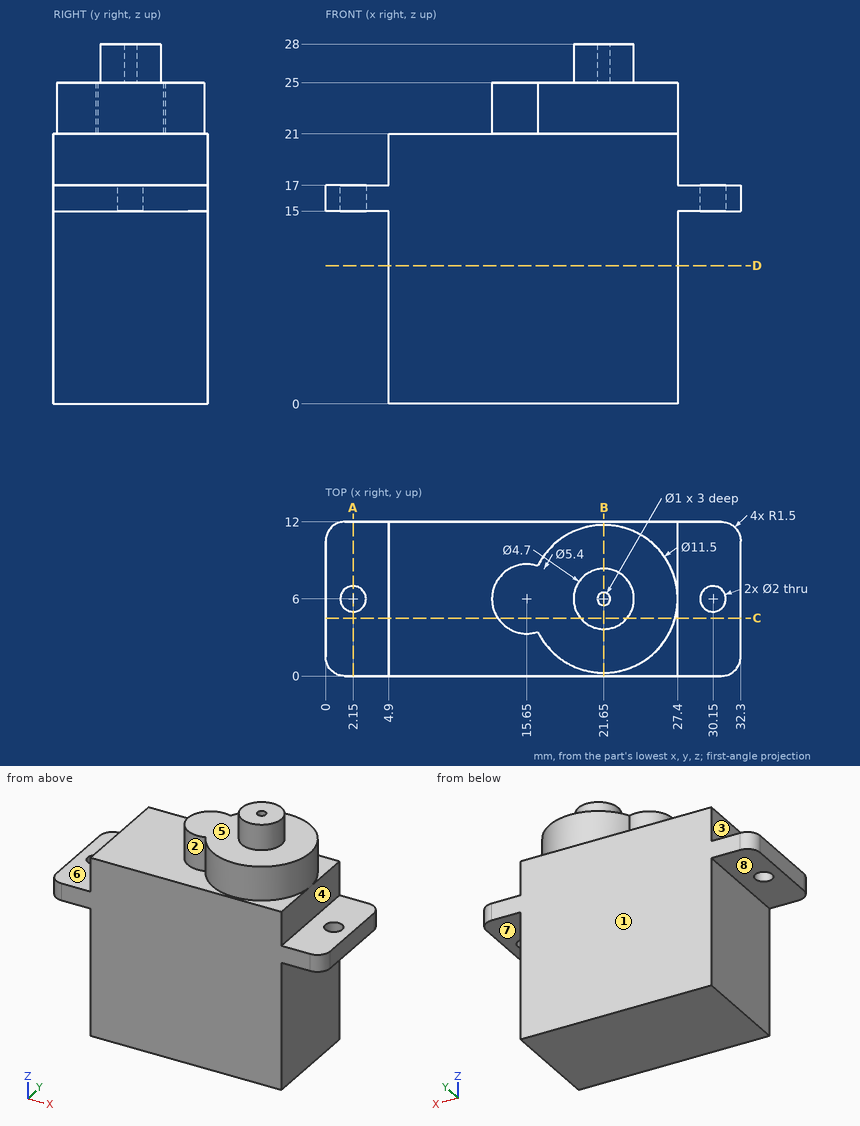
For this review, use the dimensioned drawing (mm, ordinates from the lowest corner) and the shaded views. A direction names the side the tool comes from. Give positions to 0.01 mm unless a question says otherwise; leave off trailing zeros. Write each loop counter-clockwise with the first axis right and the second up, starting at its lowest first coordinate (ties: lowest second). Pieces come first, ordered by that corner, then holes. Notation, with made-up numbers: M 31.25,28 L 69.25,28 A30 cw 69.25,64 Z; hole C 12,88.25 d8. An arc over 180 degrees is marked long. Answer as a JSON object with one key per item and string values. Group by question number.
1) We need section D-D (z = 10.75). Give the boundary of the cut face in (x, y), and give its area (3 significant figures).
2) Mouldability with a two-part tool opening along X and no side actions: class the marked faces 1, 2 and 3 as released by +X, released by -X, zero draft, split by the parting line, or undercut.
3) Clearance check with flat-ended pins moving along their axes: pin 1 Ø4 at (x, z) = (10.5, 8.5) entering from -Y; pin 2 Ø6 at (y, z) = (9, 7) entering from +X; pin 3 Ø3 at (y, z) = (8.5, 19) entering from -X; pin 4 Ø5 at (x, y) = (6, 7.5) entering from +Z. State where each tip first meets the part, or that it passes through.
4) Tool access review of the marked faces 4, 5, 6, 7 and 8: name each direction out of +Z, -Z, +X, -X, +Y, -Y from which nothing blocks a thin tool from reaching the whole face with its end or side.
5) We need section C-C (y = 4.5). Give the boundary of the cut face in (x, z) (3 decimals), and give its area (3 significant figures).
6) For line 1 along Y through (x, z) = (2.15, 15.6); line 2 along Y through (x, z) = (21.65, 25.9); line 3 along X through (y, z) = (4, 10.5), list the stretches that pass through material, from the lowest coordinate up.
7) We need section A-A (x = 2.15). Give the boundary of the cut face in (y, z), and give its area (3 significant figures).
8) We need section B-B (x = 21.65). Give the boundary of the cut face in (y, z), and give its area (3 significant figures).
Answer key:
{
 "1": {"outline": "M 4.9,0 L 27.4,0 L 27.4,12 L 4.9,12 Z", "area": "270 mm²"},
 "2": {"face 1": "zero draft", "face 2": "undercut", "face 3": "released by -X"},
 "3": {"pin 1": "stops at y = 0", "pin 2": "stops at x = 27.4", "pin 3": "stops at x = 4.9", "pin 4": "stops at z = 21"},
 "4": {"face 4": "+Z, +X, +Y, -Y", "face 5": "+Z", "face 6": "+Z, -X, +Y, -Y", "face 7": "-Z, +X, +Y, -Y", "face 8": "-Z, -X, +Y, -Y"},
 "5": {"outline": "M 0,15 L 4.9,15 L 4.9,0 L 27.4,0 L 27.4,15 L 32.3,15 L 32.3,17 L 27.4,17 L 27.4,21 L 27.201,21 L 27.201,25 L 23.459,25 L 23.459,28 L 19.841,28 L 19.841,25 L 13.405,25 L 13.405,21 L 4.9,21 L 4.9,17 L 0,17 Z", "area": "558 mm²"},
 "6": {"line 1": "y = 0 to 5, 7 to 12", "line 2": "y = 3.65 to 5.5, 6.5 to 8.35", "line 3": "x = 4.9 to 27.4"},
 "7": {"outline": "M 0,15 L 5,15 L 5,17 L 0,17 Z; M 7,15 L 12,15 L 12,17 L 7,17 Z", "area": "20.0 mm²"},
 "8": {"outline": "M 0,0 L 12,0 L 12,21 L 11.75,21 L 11.75,25 L 8.35,25 L 8.35,28 L 6.5,28 L 6.5,25 L 5.5,25 L 5.5,28 L 3.65,28 L 3.65,25 L 0.25,25 L 0.25,21 L 0,21 Z", "area": "309 mm²"}
}
